Can you work these out from the model? Positions are in its coordinate system, mm. Face numbers are marked on the shaded views. A direction names the side the tool comes from. Give positions to 0.01 mm unless a question says otherwise; leave off trailing zeros. Write each loop counter-clockwise with the first axis right and the second up, starting at its lowest first coordinate (ties: lowest second). Pieces come first, ordered by that corner, then holes. Notation, with made-up numbers: (-35.5, 46) -> (10.5, 46) arc R18 ccw to (10.5, 80) -> close; hole circle Ø6 at (30, 76). An arc over 180 degrees is marked (long way). Answer as CSV lines item,"result". Start each with the question number.
1. If we mould it in two halves opening along X, with no side actions, what happens to the marked faces 3, 4, 5 and 6? For each: pulls with the +X half, pulls with the -X half, needs draft (parallel to the pull), parting line crosses it, or undercut.
2. I'm going to push flat-ended pins straight in: P1, Ø8, axis at x = -11, z = 3, coming from the -Y side; P2, Ø2, axis at x = -10.75, z = 7.5, coming from the +Y side; P3, Ø1.2, axis at y = 1.5, z = 8, coming from the -X side; P4, Ø0.7, axis at x = 12, y = 1, coming from the +Z side. Where does each tip first touch, or does it pass through?
3. If we section it at C-C on x = 0.75: Write out the boundary of the cut face in (y, z).
4. On a 3-axis mill with a long thin cutter (end or side, diameter ignored), from which of +Z, -Z, +X, -X, +Y, -Y can I reach the whole of each face in a straight line? I mean the marked faces 1 and 2. Say none if no direction works.
5. If we section it at B-B on z = 2.25: Write out the boundary of the cut face in (x, y).
6. If we section it at A-A on y = 1.15: Write out the boundary of the cut face in (x, z).
7. I need wall thicknesses on line 1 (X direction, y = 0.85, z = 3.5); line 2 (Z direction, x = -10.75, y = 0.9); line 3 (X direction, y = 1.75, z = 7.5). Which ranges of each line are inside material? Lowest first, please. Write a range as [from, to].
```python
from build123d import *

# Parameters (mm, degrees)
SKETCH1_W           = 30
SKETCH1_H           = 24
BOSS_EXTRUDE1_DEPTH = 3
SKETCH2_R           = 1.25
CUT_EXTRUDE1_DEPTH  = 3
CUT_EXTRUDE2_DEPTH  = 3
FILLET1_R           = 5


with BuildPart() as part:
    # Sketch1 → Boss-Extrude1 (new body)
    with BuildSketch(Plane(origin=(0, 0, 0), x_dir=(1, 0, 0), z_dir=(0, 1, 0))):
        Rectangle(SKETCH1_W, SKETCH1_H)
    extrude(amount=BOSS_EXTRUDE1_DEPTH)

    # Sketch2 → Cut-Extrude1 (cut)
    with BuildSketch(Plane(origin=(0, 0, 0), x_dir=(1, 0, 0), z_dir=(0, 1, 0))):
        with Locations((-10.75, 7.5)):
            Circle(SKETCH2_R)
        with Locations((-10.75, -7.5)):
            Circle(SKETCH2_R)
        with Locations((10.75, -7.5)):
            Circle(SKETCH2_R)
        with Locations((10.75, 7.5)):
            Circle(SKETCH2_R)
    extrude(amount=CUT_EXTRUDE1_DEPTH, mode=Mode.SUBTRACT)

    # Sketch4 → Cut-Extrude2 (cut)
    with BuildSketch(Plane(origin=(0, 0, 0), x_dir=(1, 0, 0), z_dir=(0, 1, 0))):
        with BuildLine():
            Line((-10.75, 5.5), (-13, 5.5))
            Line((-13, 5.5), (-13, -5.5))
            Line((-13, -5.5), (-10.75, -5.5))
            ThreePointArc((-10.75, -5.5), (-9.335786438, -6.085786438), (-8.75, -7.5))
            Line((-8.75, -7.5), (-8.75, -10))
            Line((-8.75, -10), (8.75, -10))
            Line((8.75, -10), (8.75, -7.5))
            ThreePointArc((8.75, -7.5), (9.335786438, -6.085786438), (10.75, -5.5))
            Line((10.75, -5.5), (13, -5.5))
            Line((13, -5.5), (13, 5.5))
            Line((13, 5.5), (10.75, 5.5))
            ThreePointArc((10.75, 5.5), (9.335786438, 6.085786438), (8.75, 7.5))
            Line((8.75, 7.5), (8.75, 10))
            Line((8.75, 10), (-8.75, 10))
            Line((-8.75, 10), (-8.75, 7.5))
            ThreePointArc((-8.75, 7.5), (-9.335786438, 6.085786438), (-10.75, 5.5))
        make_face()
    extrude(amount=CUT_EXTRUDE2_DEPTH, mode=Mode.SUBTRACT)

    # Fillet1
    fillet1_edges = [part.edges().sort_by_distance(p)[0] for p in [
        (15, 1.5, 12),
        (-15, 1.5, 12),
        (-15, 1.5, -12),
        (15, 1.5, -12),
    ]]
    fillet(fillet1_edges, radius=FILLET1_R)


solid = part.part
```
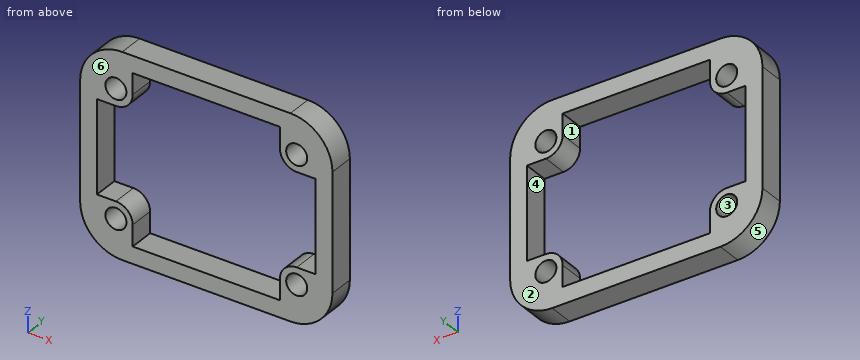
Computed values:
1,face 3,"undercut"
1,face 4,"undercut"
1,face 5,"pulls with the -X half"
1,face 6,"needs draft"
2,P1,"stops at y = 0"
2,P2,"passes through"
2,P3,"stops at x = -14.98"
2,P4,"stops at z = 11.72"
3,outline,"(0, -12) -> (3, -12) -> (3, -10) -> (0, -10) -> close; (0, 10) -> (3, 10) -> (3, 12) -> (0, 12) -> close"
4,face 1,"+Y, -Y"
4,face 2,"+Z, -Z, +X, -X, +Y"
5,outline,"(-15, 0) -> (-13, 0) -> (-13, 3) -> (-15, 3) -> close; (13, 0) -> (15, 0) -> (15, 3) -> (13, 3) -> close"
6,outline,"(-15, -7) arc R5 ccw to (-10, -12) -> (10, -12) arc R5 ccw to (15, -7) -> (15, 7) arc R5 ccw to (10, 12) -> (-10, 12) arc R5 ccw to (-15, 7) -> close; hole (-13, -5.5) -> (-10.75, -5.5) arc R2 cw to (-8.75, -7.5) -> (-8.75, -10) -> (8.75, -10) -> (8.75, -7.5) arc R2 cw to (10.75, -5.5) -> (13, -5.5) -> (13, 5.5) -> (10.75, 5.5) arc R2 cw to (8.75, 7.5) -> (8.75, 10) -> (-8.75, 10) -> (-8.75, 7.5) arc R2 cw to (-10.75, 5.5) -> (-13, 5.5) -> close; hole circle Ø2.5 at (-10.75, -7.5); hole circle Ø2.5 at (-10.75, 7.5); hole circle Ø2.5 at (10.75, -7.5); hole circle Ø2.5 at (10.75, 7.5)"
7,line 1,"x = [-15, -13], [13, 15]"
7,line 2,"z = [-11.94, -8.75], [-6.25, -5.5], [5.5, 6.25], [8.75, 11.94]"
7,line 3,"x = [-14.97, -12], [-9.5, -8.75], [8.75, 9.5], [12, 14.97]"
